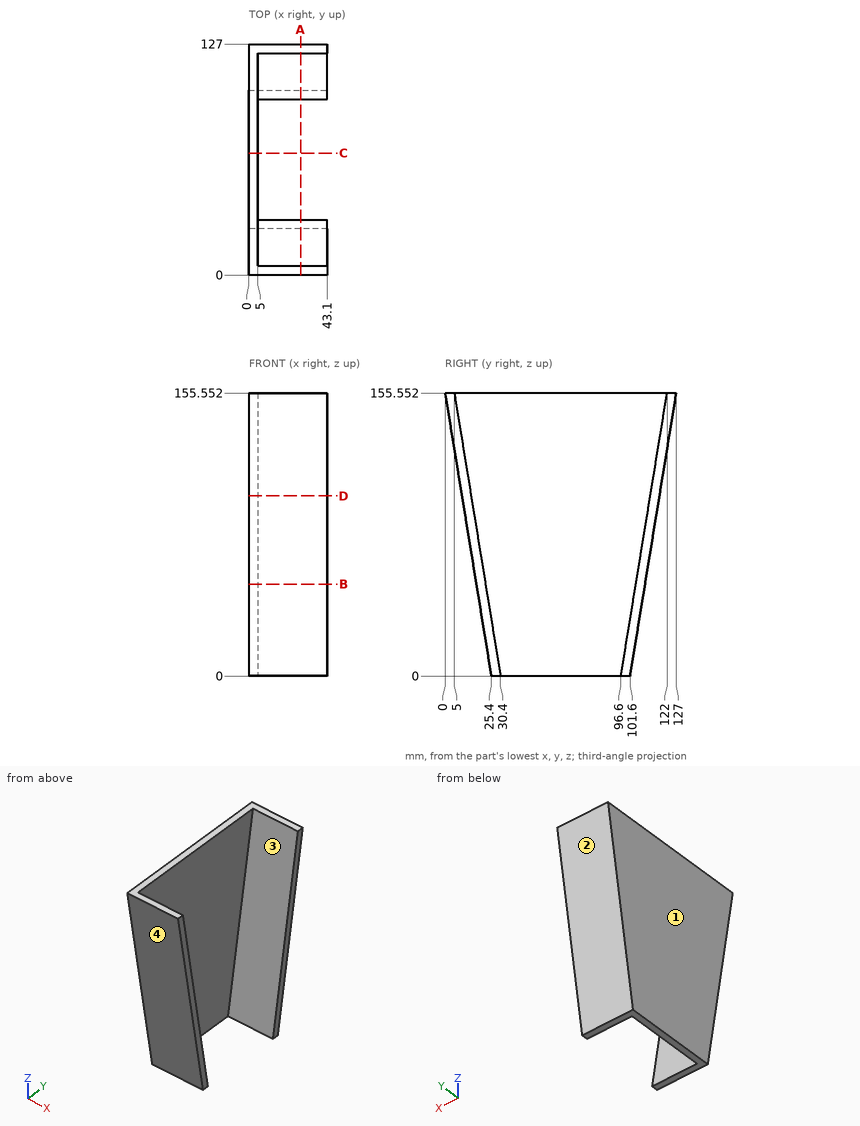
The drawing under review shows one solid part. Ordinate dimensions are in mm from its lowest x, y, z. Give positions to 0.01 mm unless a question says otherwise; leave off trailing zeros. Write each loop counter-clockwise with the first axis right and the second up, starting at its lowest first coordinate (ties: lowest second). Pieces come first, ordered by that corner, then holes. Notation, with made-up numbers: (-27, 46.5) - (-5, 46.5) arc R23 cw to (-5, 74.5) - close; hole circle Ø7 at (14, -11.5). An arc over 180 degrees is marked (long way). Answer in a Markdown table with one row per item. Add a question column.
1. We need section C-C on y = 67. Write out the cut boundary in (x, z).
2. Wall thickness on line 1 along X through (y, z) = (96, 134); line 2 along Y through (x, z) = (5.5, 124); line 3 along Y through (x, z) = (35.5, 149.5): over which ranges is each line inside the solid? List them lowest first. Write a range as [from, to].
3. Draft analysis for pull direction Y (two halves, no side actions). For the marked faces 1, 2, 3 and 4, state which applies: +Y half, -Y half, draft (parallel to the pull), parting line (faces both ways), or undercut.
4. We need section A-A on x = 28.5. Write out the cut boundary in (y, z), then the cut area to 3 significant figures.
5. We need section D-D on z = 99. Write out the cut boundary in (x, y).
6. Insertion check: P1, Ø1, axis at x = 14.5, z = 96.5, coming from the -Y side; P2, Ø4, axis at x = 33.5, z = 42, coming from the -Y side; P3, Ø10, axis at x = 8, z = 84, coming from the +Y side. Each pin has a flat end and moves straight along its axis. Give the tip position at first contact, or say it passes through.
7. We need section B-B on z = 50.5. Write out the cut boundary in (x, y).
Ans:
| question | item | result |
|---|---|---|
| 1 | outline | (0, 0) - (5, 0) - (5, 155.55) - (0, 155.55) - close |
| 2 | line 1 | x = [0, 5] |
| 2 | line 2 | y = [5.15, 10.15], [116.85, 121.85] |
| 2 | line 3 | y = [0.99, 5.99], [121.01, 126.01] |
| 3 | face 1 | draft |
| 3 | face 2 | +Y half |
| 3 | face 3 | undercut |
| 3 | face 4 | -Y half |
| 4 | outline | (0, 155.55) - (25.4, 0) - (30.4, 0) - (5, 155.55) - close; (96.6, 0) - (101.6, 0) - (127, 155.55) - (122, 155.55) - close |
| 4 | area | 1,560 mm^2 |
| 5 | outline | (0, 9.23) - (43.1, 9.23) - (43.1, 14.23) - (5, 14.23) - (5, 112.77) - (43.1, 112.77) - (43.1, 117.77) - (0, 117.77) - close |
| 6 | P1 | stops at y = 9.56 |
| 6 | P2 | stops at y = 18.22 |
| 6 | P3 | stops at y = 116.13 |
| 7 | outline | (0, 17.15) - (43.1, 17.15) - (43.1, 22.15) - (5, 22.15) - (5, 104.85) - (43.1, 104.85) - (43.1, 109.85) - (0, 109.85) - close |
